from build123d import *

# Parameters (mm, degrees)
BOSS_EXTRUDE2_DEPTH      = 85
BOSS_EXTRUDE2_DEPTH_BACK = 85
FILLET1_R                = 20
SHELL1_T                 = -5
BOSS_EXTRUDE3_DEPTH      = 5
M6_CLEARANCE_HOLE1_D     = 6.6
FILLET2_R                = 10


with BuildPart() as part:
    # Sketch4 → Boss-Extrude2 (new, two sides: drawn at the far end of the back side and taken through both)
    with BuildSketch(Plane.XY.offset(-BOSS_EXTRUDE2_DEPTH_BACK)):
        with BuildLine():
            Line((-245, 0), (-245, -10))
            ThreePointArc((-245, -10), (-239.142135624, -24.142135624), (-225, -30))
            Line((-225, -30), (-195, -30))
            ThreePointArc((-195, -30), (-189.529397686, -30.300175953), (-184.124481103, -31.197099587))
            Line((-184.124481103, -31.197099587), (-15.371875354, -68.802900413))
            ThreePointArc((-15.371875354, -68.802900413), (-9.966958771, -69.699824047), (-4.496356458, -70))
            Line((-4.496356458, -70), (170, -70))
            ThreePointArc((170, -70), (184.142135624, -64.142135624), (190, -50))
            Line((190, -50), (190, 0))
            Line((190, 0), (-245, 0))
        make_face()
    extrude(amount=BOSS_EXTRUDE2_DEPTH + BOSS_EXTRUDE2_DEPTH_BACK)

    # Fillet1
    fillet1_edges = [part.edges().sort_by_distance(p)[0] for p in [
        (-239.142135624, -24.142135624, -85),
        (-210, -30, -85),
        (-189.529397686, -30.300175953, -85),
        (-99.748178229, -50, -85),
        (-9.966958771, -69.699824047, -85),
        (-245, -5, 85),
        (-239.142135624, -24.142135624, 85),
        (-210, -30, 85),
        (-189.529397686, -30.300175953, 85),
        (-99.748178229, -50, 85),
        (-9.966958771, -69.699824047, 85),
        (82.751821771, -70, 85),
        (184.142135624, -64.142135624, 85),
        (190, -25, 85),
        (82.751821771, -70, -85),
        (184.142135624, -64.142135624, -85),
        (190, -25, -85),
        (-245, -5, -85),
    ]]
    fillet(fillet1_edges, radius=FILLET1_R)

    # Shell1
    shell1_openings = [part.faces().sort_by_distance(p)[0] for p in [
        (-27.5, 0, 0),
    ]]
    offset(amount=SHELL1_T, openings=shell1_openings, kind=Kind.INTERSECTION)

    # Sketch1 → Boss-Extrude3 (add)
    with BuildSketch(Plane(origin=(0, 0, 0), x_dir=(-1, 0, 0), z_dir=(0, 1, 0))):
        Polygon((-210, 35), (-210, -35), (-210, -105), (245, -105), (245, 105), (-210, 105), align=None)
        with BuildLine():
            Line((-170, 35), (-170, -35))
            Line((-170, -35), (-170, -65))
            ThreePointArc((-170, -65), (-165.606601718, -75.606601718), (-155, -80))
            Line((-155, -80), (215, -80))
            ThreePointArc((215, -80), (225.606601718, -75.606601718), (230, -65))
            Line((230, -65), (230, 65))
            ThreePointArc((230, 65), (225.606601718, 75.606601718), (215, 80))
            Line((215, 80), (-155, 80))
            ThreePointArc((-155, 80), (-165.606601718, 75.606601718), (-170, 65))
            Line((-170, 65), (-170, 35))
        make_face(mode=Mode.SUBTRACT)
    extrude(amount=BOSS_EXTRUDE3_DEPTH)

    # M6 Clearance Hole1 (through all)
    with Locations(Plane(origin=(0, 5, 0), x_dir=(1, 0, 0), z_dir=(0, 1, 0))):
        with Locations((165, -95), (65, -95), (-35, -95), (-135, -95), (-235, -95), (-235, 95), (-135, 95), (-35, 95), (65, 95), (165, 95)):
            Hole(M6_CLEARANCE_HOLE1_D / 2)

    # Fillet2
    fillet2_edges = [part.edges().sort_by_distance(p)[0] for p in [
        (210, 2.5, 105),
        (210, 2.5, -105),
    ]]
    fillet(fillet2_edges, radius=FILLET2_R)


solid = part.part
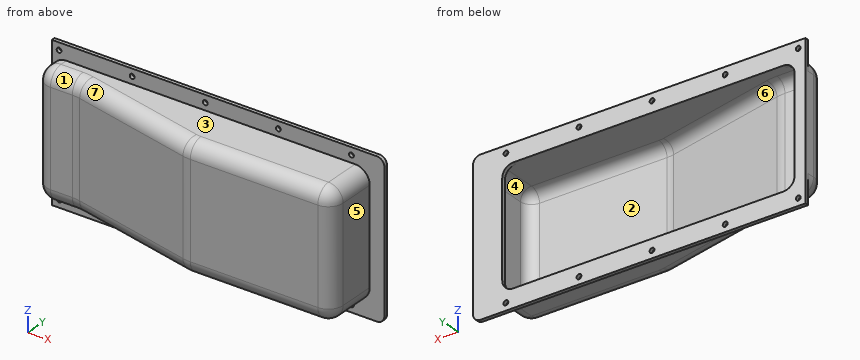
Design review of the part built by this model. Coordinates are the model's own, in mm. Face numbers are marked on the shaded views. A direction names the side the tool comes from. Give positions to 0.01 mm unless a question says otherwise; leave off trailing zeros. Order: outer loops, then holes, each group sorted by start corner. A loop starts at its lowest first (then second) coordinate and runs counter-clockwise, first axis right, second up. Notation, with made-up numbers: (51, -32) - (83, -32) arc R18 cw to (83, -25) - close; hole circle Ø5 at (-12, -37.75). An arc over 180 degrees is marked (long way). Write item = value, one per line. Start each with the question number.
Q1. We need section B-B on z = 2. State the section outline as (x, y) points, plus the area to 3 significant figures.
Q2. Clearance check with flat-ended pins moving along their axes: pin 1 Ø25 at (x, y) = (45.5, -25) entering from +Z; pin 2 Ø8.5 at (x, z) = (-135, -95) entering from +Y; pin 3 Ø8.5 at (x, z) = (65, 95) entering from -Y; pin 4 Ø10 at (x, z) = (-26.5, 22.5) entering from +Y. State where each tip first meets the part, or that it passes through.
Q3. We need section C-C on x = -206. State the section outline as (y, z) points.
Q4. To check wall thickness, follow L1, parallel to Z at x = 65, y = 1.3; L2, parallel to Z at x = -235, y = 4; L3, parallel to X at y = 3, z = -95. State the ranges of each line that lie inside material, in increasing order. Write a range as from..to.
Q5. We need section A-A on x = 133. State the section outline as (y, z) points, plus the area to 3 significant figures.
Q6. Tool access review of the marked faces 1, 2 and 3: name each direction out of +Z, -Z, +X, -X, +Y, -Y from which nothing blocks a thin tool from reaching the whole face with its end or side.
Q7. Mouldability with a two-part tool opening along Z and no side actions: class the marked faces 4, 5, 6 and 7 as released by +Z, released by -Z, zero draft, split by the parting line, or undercut.
Working result:
q1.outline = (-245, -10) arc R20 ccw to (-225, -30) - (-195, -30) arc R50 cw to (-184.12, -31.2) - (-15.37, -68.8) arc R50 ccw to (-4.5, -70) - (170, -70) arc R20 ccw to (190, -50) - (190, 0) - (210, 0) - (210, 5) - (170, 5) - (170, 0) - (185, 0) - (185, -50) arc R15 cw to (170, -65) - (-4.5, -65) arc R45 cw to (-14.28, -63.92) - (-183.04, -26.32) arc R55 ccw to (-195, -25) - (-225, -25) arc R15 cw to (-240, -10) - (-240, 0) - (-230, 0) - (-230, 5) - (-245, 5) - close
q1.area = 2,850 mm²
q2.pin_1 = 85
q2.pin_2 = 5
q2.pin_3 = 0
q2.pin_4 = -60.09
q3.outline = (-30, -65) arc R20 ccw to (-10, -85) - (0, -85) - (0, -105) - (5, -105) - (5, -80) - (-10, -80) arc R15 cw to (-25, -65) - (-25, 65) arc R15 cw to (-10, 80) - (5, 80) - (5, 105) - (0, 105) - (0, 85) - (-10, 85) arc R20 ccw to (-30, 65) - close
q4.L1 = -105..-98.3, -91.7..-80, 80..91.7, 98.3..105
q4.L2 = -105..-98.3, -91.7..91.7, 98.3..105
q4.L3 = -245..-238.3, -231.7..-138.3, -131.7..-38.3, -31.7..61.7, 68.3..161.7, 168.3..210
q5.outline = (-70, -65) arc R20 ccw to (-50, -85) - (0, -85) - (0, -105) - (5, -105) - (5, -80) - (-50, -80) arc R15 cw to (-65, -65) - (-65, 65) arc R15 cw to (-50, 80) - (5, 80) - (5, 105) - (0, 105) - (0, 85) - (-50, 85) arc R20 ccw to (-70, 65) - close
q5.area = 1,670 mm²
q6.face_1 = +Z, -X, -Y
q6.face_2 = +Y
q6.face_3 = +Z, +X, -X, -Y
q7.face_4 = undercut
q7.face_5 = zero draft
q7.face_6 = undercut
q7.face_7 = released by +Z
